Verification items for the finished model (mm, model axes). A direction names the side the tool comes from. Coordinates: 2 decimals unless noted, no trailing zeros. Use one line per item in the form item = value. Start each with the question number.
(1) Material ranges on line 1 (Y direction, x = 0, z = 11.25); line 2 (Z direction, x = 10, y = -13.5) (3 decimals); line 3 (Y direction, x = 0, z = 8.5) (3 decimals), recorded low to high. Write a range as [from, to].
(2) Gauge pin test, flat ends, axial feed: pin 1 Ø4 at (y, z) = (9, 6.5) entering from +X; pin 2 Ø5 at (x, z) = (-12, 6) entering from +Y; pin 3 Ø2 at (x, z) = (11, 10.5) entering from -Y. Record the tip position at first contact, or that the pin passes through.
(3) Mould release check, pull along Z, two halves, no side actions. Record for faces 5 (the flat face through (2, 2, 12.7)), 6 (the cylindrical face through (-15.12, -11.59, 11.09)), 7 (the cylindrical face through (-3.441, -15.497, 6.306)): released by +Z, released by -Z, zero draft, split by the parting line, or undercut.
(4) Sectioned sample at A-A (z = 1.75). Count the separate pieces of the cut face and the enclosed holes in it, and give its area (3 significant figures).
(5) Tool access check on faces 1 (the flat face through (0, -2.048, 6)), 2 (the cylindrical face through (-2.75, -12.4, 1.57)), 3 (the cylindrical face through (-1.72, -7.75, 11.13)), 4 (the flat face through (-4, 16, 3.175)). Record the directions out of +Z, -Z, +X, -X, +Y, -Y that give a thin tool (end or side, any length) a straight path to the whole face; none if there is none.
from build123d import *

# Parameters (mm, degrees)
F0_R      = 19.05
F1_DEPTH  = 3.175
F2_R      = 15.875
F3_DEPTH  = 6.35
F4_R      = 19.05
F5_DEPTH  = 3.175
F6_R      = 12.7
F6_R_2    = 7.9375
F7_DEPTH  = 3.175
F10_DEPTH = 12.7


# Not quite as in the source:
# - a pattern or mirror of a feature is missing from the dataset's text; its kind, count and spacing are read off the source's solid


with BuildPart() as f1:
    # F0 (on Top) → F1 (new body)
    with BuildSketch(Plane.XY):
        Circle(F0_R)
    extrude(amount=F1_DEPTH)

    # F2 (on face) → F3 (join)
    with BuildSketch(Plane.XY.offset(3.175)):
        Circle(F2_R)
    extrude(amount=F3_DEPTH)

    # F4 (on face) → F5 (join)
    with BuildSketch(Plane.XY.offset(9.525)):
        Circle(F4_R)
    extrude(amount=F5_DEPTH)

    # F6 (on face) → F7 (cut)
    with BuildSketch(Plane.XY.offset(12.7)):
        Circle(F6_R)
        Circle(F6_R_2, mode=Mode.SUBTRACT)
    f7 = extrude(amount=-F7_DEPTH, mode=Mode.SUBTRACT)

    # F7_copies: F7 across plane
    add(f7.mirror(Plane(origin=(0, 0, 6.35), x_dir=(-1, 0, 0), z_dir=(0, 0, -1))), mode=Mode.SUBTRACT)

    # F9 (on face) → F10 (cut, through all)
    with BuildSketch(Plane.XY.offset(12.7)):
        with BuildLine():
            Line((-1.3352941799, -2.047875), (1.3352941799, -2.047875))
            ThreePointArc((1.3352941799, -2.047875), (0, 2.44475), (-1.3352941799, -2.047875))
        make_face()
    extrude(amount=-F10_DEPTH, mode=Mode.SUBTRACT)


solid = f1.part
Answers below:
q1.line_1 = [-19.05, -12.7], [-7.94, -2.05], [2.44, 7.94], [12.7, 19.05]
q1.line_2 = [0, 3.175], [9.525, 12.7]
q1.line_3 = [-15.875, -2.048], [2.445, 15.875]
q2.pin_1 = 14.25
q2.pin_2 = 12.72
q2.pin_3 = -16.21
q3.face_5 = released by +Z
q3.face_6 = zero draft
q3.face_7 = undercut
q4.separate_pieces = 2
q4.enclosed_holes = 2
q4.area = 813 mm2
q5.face_1 = +Z, -Z
q5.face_2 = -Z
q5.face_3 = +Z
q5.face_4 = none
